Can you work these out from the model? Positions are in its coordinate system, mm. Give positions to 0.01 mm unless a question says otherwise; leave off trailing zeros. Order: outer loops, then holes, each group sorted by start corner. A loop starts at its lowest first (then second) coordinate and runs counter-clockwise, first axis right, second up. Notation, with made-up numbers: (19, -36) - (53, -36) arc R21 ccw to (53, -28) - close; hole circle Ø10 at (39, 26.25). An arc over 180 degrees is marked (long way). Use one line per item in the form item = value. Start each with the question number.
1) Suppose I cut it at B-B, the plane x = -36.5. Write out the boundary of the cut face in (y, z).
2) Please list where these lines run through material, in increasing order: probe 1 along X at (y, z) = (9.5, 0.4); probe 2 along X at (y, z) = (-15.5, 0.2); probe 3 along Y at (x, z) = (-28.5, 0.3).
3) Suppose I cut it at C-C, the plane y = 6. Write out the boundary of the cut face in (x, z).
4) Suppose I cut it at A-A, the plane z = 0.4. Write out the boundary of the cut face in (x, y), and give its area (3 significant figures).
Autodesk Inventor part; units mm, degrees
ref_plane "YZ Plane" through (0, 0, 0) normal (1, 0, 0) x (0, 1, 0)
ref_plane "XZ Plane" through (0, 0, 0) normal (0, 1, 0) x (-1, 0, 0)
ref_plane "XY Plane" through (0, 0, 0) normal (0, 0, 1) x (1, 0, 0)
sketch "Sketch1" plane through (0, 0, 0) normal (0, 0, 1) x (1, 0, 0)
  line L0 (-20.5, 22.5) -> (20.5, 22.5)
  line L1 (20.5, 22.5) -> (20.5, -22.5)
  line L2 (20.5, -22.5) -> (-20.5, -22.5)
  line L3 (-20.5, -22.5) -> (-20.5, 22.5) construction
  line L4 (-20.5, 22.5) -> (20.5, -22.5) construction
  line L5 (-20.5, -22.5) -> (-44.5, 0)
  line L6 (-44.5, 0) -> (-20.5, 22.5)
  point P0 (0, 0)
  point P1 (0, 0)
  point P2 (20.5, 0)
  dimension "d0" = 41
  dimension "d1" = 45
  dimension "d4" = 65
extrude "Plate1" add sketch "Sketch1" along normal blind 0.8
fillet "Corner Round2" radius 1 5 edges at (-20.5, -22.5, 0.4) (-44.5, 0, 0.4) (-20.5, 22.5, 0.4) (20.5, -22.5, 0.4) (20.5, 22.5, 0.4)
equation "\"d2\" = Thickness"
equation "\"BendReliefWidth\" = Thickness"
equation "\"BendReliefDepth\" = 0.5 * Thickness"
equation "\"CornerReliefSize\" = 4 * Thickness"
equation "\"MinimumRemnant\" = 2 * Thickness"
equation "\"TransitionRadius\" = BendRadius"
equation "\"JacobiRadiusSize\" = BendRadius"
equation "\"GapSize\" = Thickness"
properties part number "DSB-508 CAP house" material "Stainless Steel"
Result sheet:
q1.outline = (-7.5, 0) - (7.5, 0) - (7.5, 0.8) - (-7.5, 0.8) - close
q2.probe_1 = -34.37 to 20.5
q2.probe_2 = -27.97 to 20.5
q2.probe_3 = -15 to 15
q3.outline = (-38.1, 0) - (20.5, 0) - (20.5, 0.8) - (-38.1, 0.8) - close
q4.outline = (-43.72, -0.73) - (-20.79, -22.23) arc R1 ccw to (-20.1, -22.5) - (19.5, -22.5) arc R1 ccw to (20.5, -21.5) - (20.5, 21.5) arc R1 ccw to (19.5, 22.5) - (-20.1, 22.5) arc R1 ccw to (-20.79, 22.23) - (-43.72, 0.73) arc R1 ccw to start
q4.area = 2,380 mm²
